Geometry: final body of the model. Coordinates: model frame, mm. A direction names the side the tool comes from. Coordinates: 2 decimals unless noted, no trailing zeros. Order: outer loops, then holes, each group sorted by start corner. A loop starts at its lowest first (then second) coordinate and runs counter-clockwise, first axis right, second up. Notation, with made-up numbers: (37.25, 35.5) -> (42.25, 35.5) arc R19 ccw to (42.25, 63.5) -> close; hole circle Ø10 at (50, -7). An arc over 180 degrees is marked (long way). Use one line per item in the form item = value.
Autodesk Inventor part; units mm, degrees
ref_plane "YZ Plane" through (0, 0, 0) normal (1, 0, 0) x (0, 1, 0)
ref_plane "XZ Plane" through (0, 0, 0) normal (0, 1, 0) x (-1, 0, 0)
ref_plane "XY Plane" through (0, 0, 0) normal (0, 0, 1) x (1, 0, 0)
sketch "Sketch1" plane through (0, 0, 0) normal (0, 1, 0) x (-1, 0, 0)
  circle A0 centre (0, 0) radius 7.5
  circle A1 centre (0, 0) radius 4
  dimension "d0" = 15
  dimension "d1" = 8
extrude "Extrusion1" add sketch "Sketch1" along normal blind 24
sketch "Sketch2" plane through (0, 24, 0) normal (0, 1, 0) x (1, 0, 0)
  circle A0 centre (0, 0) radius 4
  circle A1 centre (0, 0) radius 7.5
  circle A2 centre (0, 0) radius 4.75
  dimension "d4" = 9.5
extrude "Extrusion2" cut sketch "Sketch2" against normal blind 0.2 contours A2
sketch "Sketch3" plane through (0, 0, 0) normal (0, -1, 0) x (1, 0, 0)
  circle A0 centre (0, 0) radius 4
  circle A1 centre (0, 0) radius 7.5
  circle A2 centre (0, 0) radius 4.75
  dimension "d7" = 9.5
extrude "Extrusion3" cut sketch "Sketch3" against normal blind 0.2 contours A2
fillet "Fillet1" radius 0.3 2 edges at (7.5, 0, 0) (7.5, 24, 0)
thread "Thread1"
properties part number "LM8UU" material "Stainless Steel AISI 202"
1) Material intervals for probe 1 along Z at (x, y) = (0, 23.9); probe 2 along Z at (x, y) = (-0.25, 19.5); probe 3 along Y at (x, z) = (2, -3.5), sorted ascending. Write a range as from..to.
Results found:
probe_1 = -7.42..-4.75, 4.75..7.42
probe_2 = -7.5..-3.99, 3.99..7.5
probe_3 = 0.2..23.8
2) Access query for faces 1 (the cylindrical face through (0.867, 11.835, 3.905)), 2 (the flat face through (-4, 0.2, -2)). Directions: +Z, -Z, +X, -X, +Y, -Y. A direction counts if a zero-diameter tool reaches every point of the face in a straight line with its end or side. Return the directions, or none.
Results found:
face_1 = +Y, -Y
face_2 = -Y
3) Section C-C, the plane y = 17. Output: boundary loops of the cut face in (x, z).
Results found:
outline = circle Ø15 at (0, 0); hole circle Ø8 at (0, 0)
4) Contact query for flat-ended pins moving along their axis: P1, Ø1, axis at x = -3.5, y = 6, coming from the +Z side; P2, Ø2, axis at x = 3.5, z = 0, coming from the -Y side; P3, Ø6, axis at y = 18.5, z = -4, coming from the +X side. Output: stop coordinate, or through.
Results found:
P1 = 6.87
P2 = 0.2
P3 = 7.43
5) Section B-B, the plane x = 0. Output: boundary loops of the cut face in (y, z).
Results found:
outline = (0, -7.2) arc R0.3 ccw to (0.3, -7.5) -> (23.7, -7.5) arc R0.3 ccw to (24, -7.2) -> (24, -4.75) -> (23.8, -4.75) -> (23.8, -4) -> (0.2, -4) -> (0.2, -4.75) -> (0, -4.75) -> close; (0, 4.75) -> (0.2, 4.75) -> (0.2, 4) -> (23.8, 4) -> (23.8, 4.75) -> (24, 4.75) -> (24, 7.2) arc R0.3 ccw to (23.7, 7.5) -> (0.3, 7.5) arc R0.3 ccw to (0, 7.2) -> close
6) Section A-A, the plane z = 0. Output: boundary loops of the cut face in (x, y), and give its area (3 significant figures).
Results found:
outline = (-7.5, 0.3) arc R0.3 ccw to (-7.2, 0) -> (-4.75, 0) -> (-4.75, 0.2) -> (-4, 0.2) -> (-4, 23.8) -> (-4.75, 23.8) -> (-4.75, 24) -> (-7.2, 24) arc R0.3 ccw to (-7.5, 23.7) -> close; (4, 0.2) -> (4.75, 0.2) -> (4.75, 0) -> (7.2, 0) arc R0.3 ccw to (7.5, 0.3) -> (7.5, 23.7) arc R0.3 ccw to (7.2, 24) -> (4.75, 24) -> (4.75, 23.8) -> (4, 23.8) -> close
area = 167 mm2
7) Pull-direction query (Z, two-part tool) for faces 3 (the flat face through (-4, 23.8, 2)), 4 (the flat face through (-5, 0, -1)), 5 (the cylindrical face through (7.493, 11.836, -0.33)); classes: released by +Z, released by -Z, zero draft, split by the parting line, or undercut.
Results found:
face_3 = undercut
face_4 = zero draft
face_5 = split by the parting line
